Read the model definition and answer for the solid it produces. Units are mm, in the model's axes. Face numbers are marked on the shaded views. A direction names the side the tool comes from. Coordinates: 2 decimals unless noted, no trailing zeros. Loops run counter-clockwise (first coordinate to the right, second up) from the corner with the lowest first, then second, coordinate; pieces in that order, holes last. Notation, with made-up numbers: (-32, 63) -> (15, 63) arc R13 ccw to (15, 75) -> close; hole circle Ø2 at (-26.5, 46). An arc over 180 degrees is marked (long way). Answer in a Markdown table with one row per item.
Solid Edge part; units mm, degrees
sketch "Sketch1" plane through (0, 0, 0) normal (0, -1, 0) x (1, 0, 0)
  line L0 (-56.8446, 11.9892) -> (-2.8446, 11.9892)
  line L1 (-2.8446, 11.9892) -> (-2.8446, 17.9892)
  line L2 (-2.8446, 17.9892) -> (-56.8446, 17.9892)
  line L3 (-56.8446, 17.9892) -> (-56.8446, 11.9892)
  line L4 (-62.8446, 11.9892) -> (-56.8446, 11.9892)
  line L5 (-56.8446, 11.9892) -> (-56.8446, 71.9892)
  line L6 (-56.8446, 71.9892) -> (-62.8446, 71.9892)
  line L7 (-62.8446, 71.9892) -> (-62.8446, 11.9892)
  dimension "D1" = 62.8446
  dimension "D2" = 56.8446
  dimension "D3" = 2.8446
extrude "Protrusion1" add sketch "Sketch1" along normal blind 120
sketch "Sketch2" plane through (-56.8446, -75, 44.9892) normal (1, 0, 0) x (0, 1, 0)
  circle A0 centre (55, -18) radius 5
  circle A1 centre (-25, -18) radius 5
  circle A2 centre (15, -18) radius 5
  dimension "D1" = 55
  dimension "D2" = 55
extrude "ExtrudedCutout_1" cut sketch "Sketch2" against normal blind 21.8402
sketch "Sketch3" plane through (-29.8446, -75, 17.9892) normal (0, 0, 1) x (1, 0, 0)
  circle A0 centre (-10, -25) radius 5
  circle A1 centre (-10, 59) radius 5
  dimension "D1" = 10
extrude "ExtrudedCutout_2" cut sketch "Sketch3" against normal blind 26.4448
properties material "Aluminum, 6061-T6"
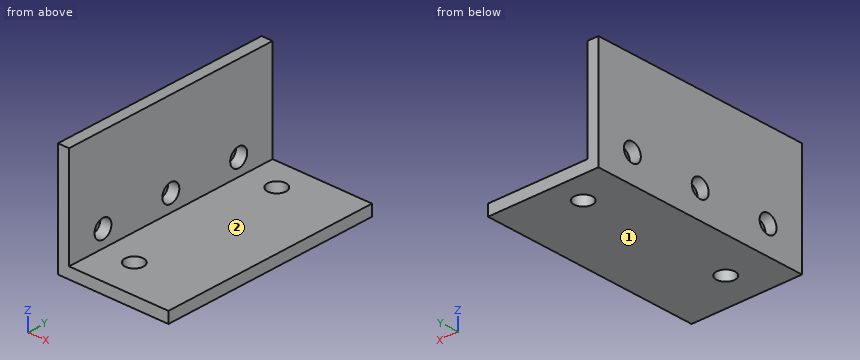
1. A cutting plane is placed at C-C on x = -55. Give the vertices of the cut face in (y, z).
A:
| item | result |
|---|---|
| outline | (-120, 11.99) -> (0, 11.99) -> (0, 17.99) -> (-120, 17.99) -> close |
2. A cutting plane is placed at D-D on z = 35. Give the vertices of the cut face in (x, y), and give its area (3 significant figures).
A:
| item | result |
|---|---|
| outline | (-62.84, -120) -> (-56.84, -120) -> (-56.84, 0) -> (-62.84, 0) -> close |
| area | 720 mm2 |
3. A tool of negligible diameter and unlimited length cuts with its end or side. For the marked faces 1 and 2, from which of +Z, -Z, +X, -X, +Y, -Y can it reach the whole face along a straight path? Write none if from no direction.
A:
| item | result |
|---|---|
| face 1 | -Z, +X, -X, +Y, -Y |
| face 2 | +Z, +X, +Y, -Y |
4. A cutting plane is placed at A-A on y = -60. Give the vertices of the cut face in (x, z), and give its area (3 significant figures).
A:
| item | result |
|---|---|
| outline | (-62.84, 11.99) -> (-2.84, 11.99) -> (-2.84, 17.99) -> (-56.84, 17.99) -> (-56.84, 21.99) -> (-62.84, 21.99) -> close; (-62.84, 31.99) -> (-56.84, 31.99) -> (-56.84, 71.99) -> (-62.84, 71.99) -> close |
| area | 624 mm2 |
5. Find the intervals of material crossed by probe 1 along Z at (x, y) = (-39, -30); probe 2 along Z at (x, y) = (-59.55, -100); probe 3 along X at (y, z) = (-93, 22.5), in increasing order.
A:
| item | result |
|---|---|
| probe 1 | z = 11.99 to 17.99 |
| probe 2 | z = 11.99 to 21.99, 31.99 to 71.99 |
| probe 3 | x = -62.84 to -56.84 |
6. Given pin 1 Ø13 at (y, z) = (-60, 26.99) entering from -X; pin 2 Ø1 at (y, z) = (-56, 25) entering from -X (1 decimal); pin 3 Ø16 at (x, y) = (-30, -83.5) entering from +Z; pin 4 Ø16 at (y, z) = (-20, 26.99) entering from +X, each flat-ended and moving along its own axis, determine where each tip first touches the part or whether it passes through.
A:
| item | result |
|---|---|
| pin 1 | stops at x = -62.84 |
| pin 2 | passes through |
| pin 3 | stops at z = 17.99 |
| pin 4 | stops at x = -56.84 |
7. A cutting plane is placed at B-B on y = -100. Give the vertices of the cut face in (x, z).
A:
| item | result |
|---|---|
| outline | (-62.84, 11.99) -> (-44.84, 11.99) -> (-44.84, 17.99) -> (-56.84, 17.99) -> (-56.84, 21.99) -> (-62.84, 21.99) -> close; (-62.84, 31.99) -> (-56.84, 31.99) -> (-56.84, 71.99) -> (-62.84, 71.99) -> close; (-34.84, 11.99) -> (-2.84, 11.99) -> (-2.84, 17.99) -> (-34.84, 17.99) -> close |
